Input: part model. Units: mm. Frame: model coordinates. A direction names the side the tool comes from. Give positions to 0.01 mm unless a question says otherwise; leave off trailing zeros. Loops run counter-clockwise (first coordinate to the right, second up) from the corner with the lowest first, then second, coordinate; pieces in that order, holes last. Notation, with made-up numbers: (89.25, 49) - (138.25, 49) arc R20 ccw to (138.25, 77) - close; hole circle Ø11 at (-37, -16). An arc over 180 degrees is marked (long way). One line per item, written item: value.
from build123d import *

# Parameters (mm, degrees)
SKETCH_1_W      = 44.5
SKETCH_1_H      = 33.5
EXTRUDE_1_DEPTH = 40
SKETCH_2_R      = 15
EXTRUDE_2_DEPTH = 12
SKETCH_3_R      = 16.5
EXTRUDE_3_DEPTH = 3
SKETCH_4_R      = 15
EXTRUDE_4_DEPTH = 20


with BuildPart() as part:
    # 草图1 → 凸台-拉伸1 (new body)
    with BuildSketch(Plane(origin=(0, 0, 0), x_dir=(1, 0, 0), z_dir=(0, 1, 0))):
        Rectangle(SKETCH_1_W, SKETCH_1_H)
    extrude(amount=EXTRUDE_1_DEPTH)

    # 草图2 → 凸台-拉伸2 (add)
    with BuildSketch(Plane(origin=(0, 0, -16.75), x_dir=(-1, 0, 0), z_dir=(0, 0, -1))):
        with Locations((0, 20)):
            Circle(SKETCH_2_R)
    extrude(amount=EXTRUDE_2_DEPTH)

    # 草图3 → 凸台-拉伸3 (add)
    with BuildSketch(Plane(origin=(0, 0, -28.75), x_dir=(-1, 0, 0), z_dir=(0, 0, -1))):
        with Locations((0, 20)):
            Circle(SKETCH_3_R)
    extrude(amount=EXTRUDE_3_DEPTH)

    # 草图4 → 凸台-拉伸4 (add)
    with BuildSketch(Plane(origin=(0, 0, -31.75), x_dir=(-1, 0, 0), z_dir=(0, 0, -1))):
        with Locations((0, 20)):
            Circle(SKETCH_4_R)
    extrude(amount=EXTRUDE_4_DEPTH)


solid = part.part
Item 1: Section A-A, the plane x = 0. Output: boundary loops of the cut face in (y, z), and give its area (3 significant figures).
Verdict:
outline: (0, -16.75) - (5, -16.75) - (5, -28.75) - (3.5, -28.75) - (3.5, -31.75) - (5, -31.75) - (5, -51.75) - (35, -51.75) - (35, -31.75) - (36.5, -31.75) - (36.5, -28.75) - (35, -28.75) - (35, -16.75) - (40, -16.75) - (40, 16.75) - (0, 16.75) - close
area: 2,400 mm^2
Item 2: Access query for faces 1 (the face through (-22.25, 20, 0)), 2 (the face through (-4, 5, -31.75)), 3 (the face through (-15, 15, -16.75)). Directions: +Z, -Z, +X, -X, +Y, -Y. A direction counts if a zero-diameter tool reaches every point of the face in a straight line with its end or side. Return the directions, or none.
Verdict:
face 1: +Z, -Z, -X, +Y, -Y
face 2: -Z
face 3: none
Item 3: Section B-B, the plane y = 20. Output: boundary loops of the cut face in (x, z), and give its area (3 significant figures).
Verdict:
outline: (-22.25, -16.75) - (-15, -16.75) - (-15, -28.75) - (-16.5, -28.75) - (-16.5, -31.75) - (-15, -31.75) - (-15, -51.75) - (15, -51.75) - (15, -31.75) - (16.5, -31.75) - (16.5, -28.75) - (15, -28.75) - (15, -16.75) - (22.25, -16.75) - (22.25, 16.75) - (-22.25, 16.75) - close
area: 2,550 mm^2
Item 4: Pin query (flat end, axial travel): P1, Ø1, axis at x = 8.5, z = -25, coming from the -Y side; P2, Ø3, axis at y = 27, z = -33, coming from the -X side. Return the tip coordinate at first contact, or that it passes through.
Verdict:
P1: stops at y = 7.31
P2: stops at x = -15.3
Item 5: Draft query along Z for faces 4 (the face through (3.252, 5.357, -22.666)), 5 (the face through (0, 20, -51.75)), 6 (the face through (-4, 5, -28.75)), 7 (the face through (0, 0, 0)). Return one class per face: pulls with the +Z half, pulls with the -Z half, needs draft (parallel to the pull), parting line crosses it, or undercut.
Verdict:
face 4: undercut
face 5: pulls with the -Z half
face 6: undercut
face 7: needs draft
Item 6: Material intervals for L1, parallel to Z at x = -11, y = 5; L2, parallel to X at y = 20.5, z = -34.5; L3, parallel to Y at x = 10, z = -19.5, sorted ascending.
Verdict:
L1: z = -16.75 to 16.75
L2: x = -14.99 to 14.99
L3: y = 8.82 to 31.18
Item 7: Section D-D, the plane x = -18. Output: boundary loops of the cut face in (y, z), and give its area (3 significant figures).
Verdict:
outline: (0, -16.75) - (40, -16.75) - (40, 16.75) - (0, 16.75) - close
area: 1,340 mm^2
Item 8: Section C-C, the plane z = -40. Output: boundary loops of the cut face in (x, y), and give its area (3 significant figures).
Verdict:
outline: circle Ø30 at (0, 20)
area: 707 mm^2
